Design review of the part built by this model. Coordinates are the model's own, in mm. A direction names the side the tool comes from. Coordinates: 2 decimals unless noted, no trailing zeros. Order: outer loops, then holes, each group sorted by start corner. A loop starts at its lowest first (then second) coordinate and runs counter-clockwise, first axis right, second up. Notation, with made-up numbers: M 4,88.5 L 47,88.5 A25 cw 47,111.5 Z; hole C 6.25,82 d6. An arc over 180 degrees is marked long. Use CSV: the item, a comma, the result in double quotes.
Autodesk Inventor part; units mm, degrees
ref_plane "Work Plane3" through (0, 0, 0) normal (0, 0, 1) x (1, 0, 0)
ref_plane "Work Plane4" through (0, 0, 19.05) normal (0, 0, 1) x (1, 0, 0)
ref_plane "Work Plane1" through (-127, 50.8, 9.525) normal (0, 0, 1) x (1, 0, 0)
sketch "Sketch1" plane through (0, 0, 0) normal (0, 0, 1) x (1, 0, 0)
  line L0 (-127, -76.2) -> (127, -76.2)
  line L1 (127, -76.2) -> (127, 76.2)
  line L2 (127, 76.2) -> (-127, 76.2)
  line L3 (-127, 76.2) -> (-127, -76.2)
  line L4 (-127, -76.2) -> (127, 76.2) construction
  line L5 (127, -76.2) -> (-127, 76.2) construction
  point P0 (0, 0)
  dimension "d0" = 254
  dimension "d1" = 152.4
extrude "Extrusion1" add sketch "Sketch1" along normal mid plane 38.1
sketch "Sketch10" plane through (0, 0, 19.05) normal (0, 0, 1) x (1, 0, 0)
  line L0 (-127, -13.335) -> (127, -13.335)
  line L1 (127, -13.335) -> (127, 13.335)
  line L2 (127, 13.335) -> (-127, 13.335)
  line L3 (-127, 13.335) -> (-127, -13.335)
  line L4 (-127, -13.335) -> (127, 13.335) construction
  line L5 (127, -13.335) -> (-127, 13.335) construction
  line L6 (-127, 76.2) -> (-127, -76.2)
  point P0 (0, 0)
  dimension "d71" = 26.67
extrude "Extrusion7" cut sketch "Sketch10" against normal blind 20.32
ref_plane "Work Plane3" through (0, 0, 0) normal (0, 0, 1) x (1, 0, 0)
ref_plane "Work Plane4" through (0, 0, 19.05) normal (0, 0, 1) x (1, 0, 0)
sketch "Sketch11" plane through (0, 0, -1.27) normal (0, 0, 1) x (1, 0, 0)
  line L0 (-127, -7.62) -> (127, -7.62)
  line L1 (127, -7.62) -> (127, 7.62)
  line L2 (127, 7.62) -> (-127, 7.62)
  line L3 (-127, 7.62) -> (-127, -7.62)
  line L4 (-127, -7.62) -> (127, 7.62) construction
  line L5 (127, -7.62) -> (-127, 7.62) construction
  line L6 (-127, 76.2) -> (-127, 13.335)
  point P0 (0, 0)
  dimension "d75" = 15.24
extrude "Extrusion8" cut sketch "Sketch11" against normal blind 12.7
sketch "Sketch12" plane through (0, 0, 19.05) normal (0, 0, 1) x (1, 0, 0)
  line L0 (-127, 76.2) -> (-127, 13.335)
  line L1 (-127, 63.5) -> (76.2, 63.5)
  line L2 (76.2, 63.5) -> (76.2, -63.5)
  line L3 (76.2, -63.5) -> (-127, -63.5)
  line L4 (-127, -63.5) -> (-127, 63.5)
  line L5 (127, 76.2) -> (-127, 76.2)
  line L6 (-127, -76.2) -> (127, -76.2)
  point P0 (0, 0)
  dimension "d78" = 12.7
  dimension "d79" = 12.7
  dimension "d80" = 203.2
extrude "Extrusion9" cut sketch "Sketch12" against normal blind 13.97
sketch "Sketch3" plane through (0, 0, 19.05) normal (0, 0, 1) x (1, 0, 0)
  line L0 (-76.2, -12.7) -> (76.2, -12.7)
  line L1 (76.2, -12.7) -> (76.2, 12.7)
  line L2 (76.2, 12.7) -> (-76.2, 12.7)
  line L3 (-76.2, 12.7) -> (-76.2, -12.7)
  line L4 (-76.2, -12.7) -> (76.2, 12.7) construction
  line L5 (76.2, -12.7) -> (-76.2, 12.7) construction
  point P0 (0, 0)
  dimension "d7" = 25.4
  dimension "d19" = 152.4
sketch "Sketch8" plane through (0, 0, 19.05) normal (0, 0, 1) x (1, 0, 0)
  line L0 (-76.2, -12.7) -> (-76.2, 12.7)
  line L1 (-76.2, 0) -> (38.1, 0)
  line L2 (38.1, 0) -> (38.1, 38.1)
  line L3 (38.1, 38.1) -> (-76.2, 38.1)
  line L4 (-76.2, 38.1) -> (-76.2, 0)
  line L5 (38.1, 0) -> (38.1, -38.1)
  line L6 (38.1, -38.1) -> (-76.2, -38.1)
  line L7 (-76.2, -38.1) -> (-76.2, 0)
  point P0 (0, 0)
  dimension "d51" = 114.3
  dimension "d52" = 38.1
sketch "Sketch9" plane through (0, 0, 19.05) normal (0, 0, 1) x (1, 0, 0)
  line L0 (-127, 76.2) -> (-127, -76.2) construction
  line L1 (-127, -57.15) -> (127, -57.15) construction
  line L2 (127, 76.2) -> (127, -76.2) construction
  line L3 (-127, -57.15) -> (-127, -44.4609) construction
  point P0 (0, 0)
  point P1 (-127, 76.2)
  point P2 (-76.2, 38.1)
  point P3 (-101.6, -57.15)
  point P4 (-76.2, -57.15)
  point P5 (-50.8, -57.15)
  point P6 (-25.4, -57.15)
  point P7 (0, -57.15)
  point P8 (-101.6, -146.05)
  point P9 (-76.2, -146.05)
  point P10 (-50.8, -146.05)
  point P11 (-25.4, -146.05)
  point P12 (0, -146.05)
  point P13 (-101.6, -234.95)
  point P14 (-76.2, -234.95)
  point P15 (-50.8, -234.95)
  point P16 (-25.4, -234.95)
  point P17 (0, -234.95)
  point P18 (-101.6, -323.85)
  point P19 (-76.2, -323.85)
  point P20 (-50.8, -323.85)
  point P21 (-25.4, -323.85)
  point P22 (0, -323.85)
  point P23 (-127, -76.2)
  dimension "d55" = 25.4
  dimension "d58" = 25.4
  dimension "d61" = 88.9
properties part number "pistonHousing-8-in" material "PET Plastic"
(1) Add section D-D on x = -40. State the section outline as (y, z) points (3 decimals), and give its area (3 significant figures).
The answers:
outline,"M -76.2,-19.05 L 76.2,-19.05 L 76.2,19.05 L 63.5,19.05 L 63.5,5.08 L 13.335,5.08 L 13.335,-1.27 L 7.62,-1.27 L 7.62,-13.97 L -7.62,-13.97 L -7.62,-1.27 L -13.335,-1.27 L -13.335,5.08 L -63.5,5.08 L -63.5,19.05 L -76.2,19.05 Z"
area,"3,670 mm2"
(2) The part is to be moulded in two halves that separate along Y. For faces 4 (the face through (26.4, -13.335, 4.5)), 5 (the face through (2, 76.2, 0)), 6 (the face through (-127, 1, -17)), 7 (the face through (-2, -7.62, -8)), say which applies: pulls with the +Y half, pulls with the -Y half, needs draft (parallel to the pull), parting line crosses it, or undercut.
The answers:
face 4,"undercut"
face 5,"pulls with the +Y half"
face 6,"needs draft"
face 7,"undercut"
(3) Clearance check with flat-ended pins moving along their axes: P1, Ø7, axis at y = 31.5, z = 13.5, coming from the -X side; P2, Ø3, axis at x = -15, y = 9.5, coming from the +Z side; P3, Ø7.5, axis at x = 31, y = -2.5, coming from the +Z side. State where each tip first meets the part, or that it passes through.
The answers:
P1,"stops at x = 76.2"
P2,"stops at z = -1.27"
P3,"stops at z = -13.97"
(4) For faces 1 (the face through (-2, -76.2, 0)), 2 (the face through (2, 7.62, -8)), 3 (the face through (-27, 63.5, 12)), list the 3-axis set-ups (+Z, -Z, +X, -X, +Y, -Y) from which the entire face can be reached by the end or side of a thin tool; tool diameter is ignored.
The answers:
face 1,"+Z, -Z, +X, -X, -Y"
face 2,"+Z, +X, -X"
face 3,"+Z, -X"
(5) Add section C-C on y = 33. State the section outline as (x, z) points.
The answers:
outline,"M -127,-19.05 L 127,-19.05 L 127,19.05 L 76.2,19.05 L 76.2,5.08 L -127,5.08 Z"
(6) Wall thickness on probe 1 along Y at (x, z) = (42.5, -1.5); probe 2 along Y at (x, z) = (99, 12) (3 decimals); probe 3 along X at (y, z) = (55.5, 9): over which ranges is each line inside the solid? List them lowest first.
The answers:
probe 1,"y = -76.2 to -7.62, 7.62 to 76.2"
probe 2,"y = -76.2 to -13.335, 13.335 to 76.2"
probe 3,"x = 76.2 to 127"
(7) Add section A-A on z = -6. State the section outline as (x, y) points, and give its area (3 significant figures).
The answers:
outline,"M -127,-76.2 L 127,-76.2 L 127,-7.62 L -127,-7.62 Z; M -127,7.62 L 127,7.62 L 127,76.2 L -127,76.2 Z"
area,"34,800 mm2"
(8) Add section B-B on x = 84.5. State the section outline as (y, z) points (3 decimals).
The answers:
outline,"M -76.2,-19.05 L 76.2,-19.05 L 76.2,19.05 L 13.335,19.05 L 13.335,-1.27 L 7.62,-1.27 L 7.62,-13.97 L -7.62,-13.97 L -7.62,-1.27 L -13.335,-1.27 L -13.335,19.05 L -76.2,19.05 Z"
